Autodesk Inventor part; units mm, degrees
ref_plane "YZ Plane" through (0, 0, 0) normal (1, 0, 0) x (0, 1, 0)
ref_plane "XZ Plane" through (0, 0, 0) normal (0, 1, 0) x (-1, 0, 0)
ref_plane "XY Plane" through (0, 0, 0) normal (0, 0, 1) x (1, 0, 0)
sketch "Sketch1" plane through (0, 0, 0) normal (0, 0, 1) x (1, 0, 0)
  line L0 (-16.3829, -30.3318) -> (-62.1829, -30.3318)
  line L1 (-64.1829, -80.1318) -> (-14.3829, -80.1318) construction
  line L2 (35.6171, -80.1318) -> (-104.3829, -80.1318)
  line L3 (-104.3829, -80.1318) -> (-104.3829, -30.3318)
  line L4 (-104.3829, -30.3318) -> (35.6171, -30.3318)
  line L5 (35.6171, -30.3318) -> (35.6171, -80.1318)
  line L6 (-14.3829, -78.1318) -> (-14.3829, -32.3318)
  circle A0 centre (-19.2829, -75.2318) radius 1.4
  circle A1 centre (-59.2829, -75.2318) radius 1.4
  circle A2 centre (-19.2829, -35.2318) radius 1.4
  circle A3 centre (-59.2829, -35.2318) radius 1.4
extrude "Extrusion1" add sketch "Sketch1" along normal blind 4.5
sketch "Sketch4" plane through (0, 0, 4.5) normal (0, 0, 1) x (1, 0, 0)
  circle A0 centre (10.7171, -55.2318) radius 16.9 construction
  circle A1 centre (-9.2829, -35.2318) radius 1.45
  circle A2 centre (30.7171, -35.2318) radius 1.45
  arc A3 (-9.2829, -73.8318) -> (-9.2829, -76.6318) centre (-9.2829, -75.2318) ccw
  arc A4 (-9.2829, -73.8318) -> (-9.2829, -76.6318) centre (-9.2829, -75.2318) ccw
  arc A5 (30.7171, -76.6318) -> (30.7171, -73.8318) centre (30.7171, -75.2318) ccw
  circle A6 centre (30.7171, -75.2318) radius 1.4
  circle A7 centre (30.7171, -35.2318) radius 1.4
  circle A8 centre (-9.2829, -75.2318) radius 1.4
  circle A9 centre (-9.2829, -35.2318) radius 1.4
  circle A10 centre (10.7171, -55.2318) radius 17.5
  point P0 (0, 0)
  dimension "d44" = 2.8
  dimension "d45" = 2.8
  dimension "d46" = 2.8
  dimension "d47" = 2.8
  dimension "d48" = 35
extrude "Extrusion3" cut sketch "Sketch4" against normal through all contours A8 A3 | A6 A5 | A7 | A9 | A10
sketch "Sketch3" plane through (0, 0, 4.5) normal (0, 0, 1) x (1, 0, 0)
  circle A0 centre (-9.2829, -35.2318) radius 1.4
  circle A1 centre (-9.2829, -75.2318) radius 1.4
  circle A2 centre (30.7171, -75.2318) radius 1.4
  circle A3 centre (10.7171, -55.2318) radius 17.5
  circle A4 centre (30.7171, -35.2318) radius 1.4
  circle A5 centre (-59.2829, -35.2318) radius 1.4
  circle A6 centre (-19.2829, -35.2318) radius 1.4
  circle A7 centre (-59.2829, -75.2318) radius 1.4
  circle A8 centre (-19.2829, -75.2318) radius 1.4
  line L0 (-104.3829, -80.1318) -> (35.6171, -80.1318)
  line L1 (35.6171, -80.1318) -> (35.6171, -30.3318)
  line L2 (35.6171, -30.3318) -> (-104.3829, -30.3318)
  line L3 (-104.3829, -30.3318) -> (-104.3829, -80.1318)
  circle A9 centre (30.7171, -75.2318) radius 3
  circle A10 centre (-9.2829, -75.2318) radius 3
  circle A11 centre (-19.2829, -75.2318) radius 3
  circle A12 centre (-59.2829, -75.2318) radius 3
  circle A13 centre (30.7171, -35.2318) radius 3
  circle A14 centre (-9.2829, -35.2318) radius 3
  circle A15 centre (-19.2829, -35.2318) radius 3
  circle A16 centre (-59.2829, -35.2318) radius 3
  dimension "d51" = 1.6
  dimension "d52" = 1.6
  dimension "d53" = 1.6
  dimension "d54" = 1.6
  dimension "d55" = 1.6
  dimension "d56" = 1.6
  dimension "d57" = 1.6
  dimension "d58" = 1.6
extrude "Extrusion2" cut sketch "Sketch3" against normal blind 3.2 contours A9 | A10 | A11 | A12 | A13 | A14 | A15 | A16
fillet "Fillet1" radius 5 4 edges at (35.6171, -30.3318, 2.25) (-104.3829, -30.3318, 2.25) (-104.3829, -80.1318, 2.25) (35.6171, -80.1318, 2.25)
equation "\"d44\" = d40"
equation "\"d45\" = d40"
equation "\"d46\" = d40"
equation "\"d47\" = d40"
equation "\"d52\" = d51"
equation "\"d53\" = d51"
equation "\"d54\" = d51"
equation "\"d55\" = d51"
equation "\"d56\" = d51"
equation "\"d57\" = d51"
equation "\"d58\" = d51"
equation "\"d41\" = d40"
equation "\"d42\" = d40"
equation "\"d43\" = d40"
properties part number "30_Smartphone_Holder"
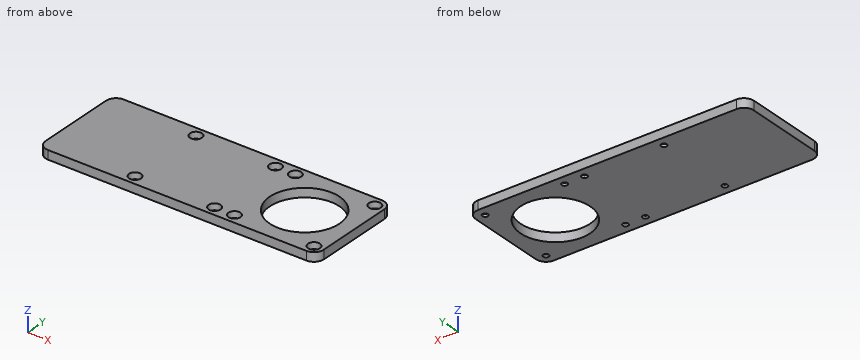
For this review, take the finished solid that the model builds, in its own axes (mm). Round coordinates to 2 decimals unless told otherwise and drop trailing zeros. Write each loop counter-clockwise with the first axis right and the second up, starting at its lowest first coordinate (ties: lowest second). Pieces come first, ordered by that corner, then holes. Notation, with made-up numbers: (76, 14.25) - (93, 14.25) arc R27 ccw to (93, 31.25) - close; hole circle Ø7 at (-0.5, 77). An arc over 180 degrees is marked (long way). Answer as CSV lines item,"result". Start each with the question number.
(1) Add section B-B, the plane x = -3.5. State the section outline as (y, z) points.
(2) For pin 1 (1.7 mm diameter, centred on x = -19.28, y = -35.23, fed in from +Z); pin 2 (3 mm diameter, centred on x = 31, y = -34.5, fed in from +Z), all flat-tipped, find the tip position at first contact; note any pin that passes through.
(3) Add section A-A, the plane y = -43. State the section outline as (x, z) points, plus the area to 3 significant figures.
(4) Add section C-C, the plane z = 3. State how many separate pieces and enclosed holes the cut face has, plus the area to 3 significant figures.
(5) For line 1 (Y direction, x = -19.5, z = 2.55); line 2 (X direction, y = -59.5, z = 4.1); line 3 (Y direction, x = 11.5, z = 0.85), list the stretches that pass through material, from the lowest coordinate up.
From the geometry:
1,outline,"(-80.13, 0) - (-65.44, 0) - (-65.44, 4.5) - (-80.13, 4.5) - close; (-45.03, 0) - (-30.33, 0) - (-30.33, 4.5) - (-45.03, 4.5) - close"
2,pin 1,"passes through"
2,pin 2,"stops at z = 1.3"
3,outline,"(-104.38, 0) - (-1.8, 0) - (-1.8, 4.5) - (-104.38, 4.5) - close; (23.23, 0) - (35.62, 0) - (35.62, 4.5) - (23.23, 4.5) - close"
3,area,"517 mm²"
4,separate pieces,"1"
4,enclosed holes,"9"
4,area,"5,760 mm²"
5,line 1,"y = -80.13 to -78.22, -72.24 to -38.22, -32.24 to -30.33"
5,line 2,"x = -104.38 to -6.25, 27.69 to 35.62"
5,line 3,"y = -80.13 to -72.71, -37.75 to -30.33"
